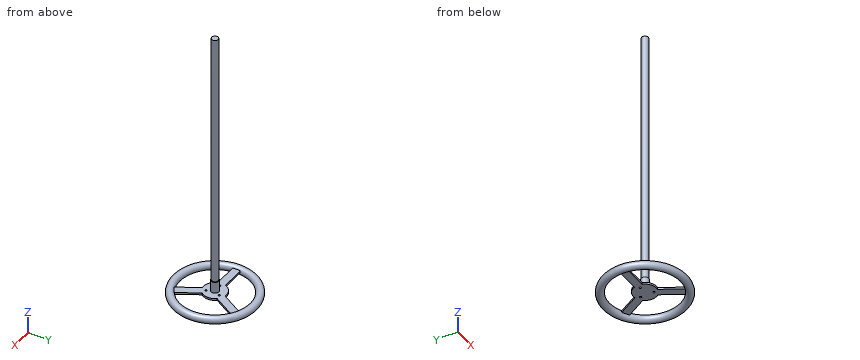
```python
from build123d import *

# Parameters (mm, degrees)
SKETCH3_R           = 30
SKETCH3_R_2         = 2.5
BOSS_EXTRUDE1_DEPTH = 5
SKETCH4_R           = 8.35
BOSS_EXTRUDE2_DEPTH = 700
SKETCH6_R           = 10
BOSS_EXTRUDE3_DEPTH = 30
BOSS_EXTRUDE4_DEPTH = 5
SKETCH11_R          = 10


with BuildPart() as part:
    # Sketch3 → Boss-Extrude1 (new body)
    with BuildSketch(Plane.XY):
        Circle(SKETCH3_R)
        with Locations((-20, 0)):
            Circle(SKETCH3_R_2, mode=Mode.SUBTRACT)
        with Locations((10, 17.320508076)):
            Circle(SKETCH3_R_2, mode=Mode.SUBTRACT)
        with Locations((10, -17.320508076)):
            Circle(SKETCH3_R_2, mode=Mode.SUBTRACT)
    extrude(amount=BOSS_EXTRUDE1_DEPTH)

    # Sketch4 → Boss-Extrude2 (add)
    with BuildSketch(Plane.XY.offset(5)):
        Circle(SKETCH4_R)
    extrude(amount=BOSS_EXTRUDE2_DEPTH)

    # Sketch6 → Boss-Extrude3 (add)
    with BuildSketch(Plane.XY.offset(5)):
        Circle(SKETCH6_R)
    extrude(amount=BOSS_EXTRUDE3_DEPTH)

    # Sketch8 → Boss-Extrude4 (add)
    with BuildSketch(Plane(origin=(0, 0, 0), x_dir=(-1, 0, 0), z_dir=(0, 0, -1))):
        with BuildLine():
            Line((-58.409625893, 81.168439698), (-22.802389662, 19.494897428))
            ThreePointArc((-22.802389662, 19.494897428), (-15, 25.980762114), (-5.481881586, 29.494897428))
            Line((-5.481881586, 29.494897428), (-41.089117817, 91.168439698))
            ThreePointArc((-41.089117817, 91.168439698), (-50, 86.602540378), (-58.409625893, 81.168439698))
        make_face()
        with BuildLine():
            Line((28.284271247, -10), (99.498743711, -10))
            ThreePointArc((99.498743711, -10), (99.874607311, -5.006277506), (100, 0))
            ThreePointArc((100, 0), (99.874607311, 5.006277506), (99.498743711, 10))
            Line((99.498743711, 10), (28.284271247, 10))
            ThreePointArc((28.284271247, 10), (29.56795679, 5.073059362), (30, 0))
            ThreePointArc((30, 0), (29.56795679, -5.073059362), (28.284271247, -10))
        make_face()
        with BuildLine():
            ThreePointArc((-58.409625893, -81.168439698), (-50, -86.602540378), (-41.089117817, -91.168439698))
            Line((-41.089117817, -91.168439698), (-5.481881586, -29.494897428))
            ThreePointArc((-5.481881586, -29.494897428), (-15, -25.980762114), (-22.802389662, -19.494897428))
            Line((-22.802389662, -19.494897428), (-58.409625893, -81.168439698))
        make_face()
    extrude(amount=-BOSS_EXTRUDE4_DEPTH)

    # Sweep1: sweep along a path in Sketch10
    with BuildLine(Plane(origin=(0, 0, 0), x_dir=(-1, 0, 0), z_dir=(0, 0, -1))) as sweep1_path:
        CenterArc((0, 0), 100, 0, 360)
    # Sketch11 → Sweep1 (sweep)
    with BuildSketch(Plane(origin=(0, 0, 0), x_dir=(1, 0, 0), z_dir=(0, 1, 0))):
        with Locations((100, 0)):
            Circle(SKETCH11_R)
    sweep(path=sweep1_path.line)


solid = part.part
```
Work out the finished part from the listing and answer in its coordinate system (mm). Round coordinates to 2 decimals unless told otherwise and drop trailing zeros. Write each loop counter-clockwise with the first axis right and the second up, starting at its lowest first coordinate (ties: lowest second). Pieces come first, ordered by that corner, then holes.
1) A cutting plane is placed at A-A on y = -50. Give the number of separate pieces and of enclosed holes in the cut face, and give its area (3 significant figures).
2) Flat-ended cylindrical pins translate along their axes: P1, Ø4, axis at y = 0, z = 119.5, coming from the +X side; P2, Ø4, axis at x = -47.5, z = 2.5, coming from the +Y side; P3, Ø6, axis at x = 10, y = 17.32, coming from the +Z side; P4, Ø4, axis at x = 10, y = -17.32, coming from the +Z side. Find the tip coordinate at first contact, or state that the pin passes through.
3) Consider probe 1 along Y at (x, z) = (10, 1); probe 2 along Y at (x, z) = (-20, 3.6); probe 3 along Y at (x, z) = (10, 1.55). Determine where each line is inside the solid, lowest interval first.
4) A cutting plane is placed at B-B on z = 617.5. Determine the outline of the cut face in (x, y), and give its area (3 significant figures).
Entries:
1. separate pieces: 3
1. enclosed holes: 0
1. area: 842 mm2
2. P1: stops at x = 8.35
2. P2: stops at y = 99.91
2. P3: stops at z = 5
2. P4: passes through
3. probe 1: y = -109.49 to -89.49, -37.32 to -19.82, -14.82 to 14.82, 19.82 to 37.32, 89.49 to 109.49
3. probe 2: y = -107.48 to -88.44, -22.36 to -2.5, 2.5 to 22.36, 88.44 to 107.48
3. probe 3: y = -109.42 to -89.56, -37.32 to -19.82, -14.82 to 14.82, 19.82 to 37.32, 89.56 to 109.42
4. outline: circle Ø16.7 at (0, 0)
4. area: 219 mm2
